Read the model definition and answer for the solid it produces. Units are mm, in the model's axes. A direction names the side the tool comes from. Coordinates: 2 decimals unless noted, no trailing zeros. Order: outer loops, then holes, each group sorted by start corner. A loop starts at its lowest first (then second) coordinate and runs counter-clockwise, first axis right, second up. Notation, with made-up numbers: M -4.5,82.25 L 46.5,82.25 A13 cw 46.5,101.25 Z; hole C 0.25,77.5 d6. An arc over 180 degrees is marked long. Write each question's results on one line, items separated by ' | '.
```python
from build123d import *

# Parameters (mm, degrees)
F1_DEPTH     = 25.4
F3_DEPTH     = 25.401
F4_T1_DEPTH  = 75.1590131963
F4_T6_DEPTH  = 127
F4_T11_DEPTH = 127
F4_T16_DEPTH = 127
F4_T21_DEPTH = 127
F4_T26_DEPTH = 121.344223221
F4_T31_DEPTH = 121.344223221
F4_T36_DEPTH = 121.344223221
F4_T41_DEPTH = 121.344223221
F4_T47_DEPTH = 121.344223221
F4_T51_DEPTH = 127
F4_T58_DEPTH = 127
F4_T62_DEPTH = 121.344223221
F4_T69_DEPTH = 121.344223221
F4_T73_DEPTH = 127
F4_T80_DEPTH = 127
F4_T84_DEPTH = 121.344223221


# Not quite as in the source:
# - a fillet or chamfer that OpenCascade refuses, or shapes differently, is made with other operations: its cross-section is extruded or revolved along the edge and cut away or added


with BuildPart() as f1:
    # F0 (on Front) → F1 (new body)
    with BuildSketch(Plane.XZ):
        Polygon((4.8083475167, 0), (0, 0), (-4.8083475167, 0), (-50.8, 63.5), (-68.9793676138, 63.5), (-12.7, -14.2040973853), (-12.7, -115.8040973853), (0, -115.8040973853), (12.7, -115.8040973853), (12.7, -14.2040973853), (68.9793676138, 63.5), (50.8, 63.5), align=None)
    extrude(amount=F1_DEPTH)

    # F2 (on face) → F3 (cut, through all)
    with BuildSketch(Plane(origin=(0, 0, 0), x_dir=(-1, 0, 0), z_dir=(0, 1, 0))):
        with BuildLine():
            ThreePointArc((-46.3238090676, 51.3453096211), (-51.0863090676, 56.1078096211), (-55.8488090676, 51.3453096211))
            Line((-55.8488090676, 51.3453096211), (-46.3238090676, 51.3453096211))
        make_face()
        with BuildLine():
            Line((-46.3238090676, 51.3453096211), (-55.8488090676, 51.3453096211))
            ThreePointArc((-55.8488090676, 51.3453096211), (-51.0863090676, 46.5828096211), (-46.3238090676, 51.3453096211))
        make_face()
        with BuildLine():
            ThreePointArc((55.8488090676, 51.3453096211), (51.0863090676, 56.1078096211), (46.3238090676, 51.3453096211))
            Line((46.3238090676, 51.3453096211), (55.8488090676, 51.3453096211))
        make_face()
        with BuildLine():
            Line((55.8488090676, 51.3453096211), (46.3238090676, 51.3453096211))
            ThreePointArc((46.3238090676, 51.3453096211), (51.0863090676, 46.5828096211), (55.8488090676, 51.3453096211))
        make_face()
    extrude(amount=-F3_DEPTH, mode=Mode.SUBTRACT)

    # F4: fillet of radius 5.08 on 10 edges, made by hand

    # F4_s2 → F4_t1 (cut)
    with BuildSketch(Plane.XZ.offset(-24.8795065982)):
        with BuildLine():
            ThreePointArc((-63.1417971968, 55.440152148), (-63.552165901, 60.7296290732), (-59.0275649745, 63.5))
            Line((-59.0275649745, 63.5), (-68.9793676138, 63.5))
            Line((-68.9793676138, 63.5), (-63.1417971968, 55.440152148))
        make_face()
        with BuildLine():
            ThreePointArc((63.1417971968, 55.440152148), (63.552165901, 60.7296290732), (59.0275649745, 63.5))
            Line((59.0275649745, 63.5), (68.9793676138, 63.5))
            Line((68.9793676138, 63.5), (63.1417971968, 55.440152148))
        make_face()
    extrude(amount=F4_T1_DEPTH, mode=Mode.SUBTRACT)


with BuildPart() as f4_tool4:
    # F4_s5 → F4_t6 (new body)
    with BuildSketch(Plane.XY.offset(-128.5040973853)):
        with BuildLine():
            ThreePointArc((12.7, -5.08), (11.2121024484, -1.4878975516), (7.62, 0))
            Line((7.62, 0), (12.7, 0))
            Line((12.7, 0), (12.7, -5.08))
        make_face()
    extrude(amount=F4_T6_DEPTH)

    split(bisect_by=Plane(origin=(15.0780779602, 0, -10.9207200262), x_dir=(0, 1, 0), z_dir=(0.8098882327, 0, -0.5865842228)), keep=Keep.TOP)


with BuildPart() as f1_1:
    add(f1.part)

    # F4_t3: cut F4_tool4
    add(f4_tool4.part, mode=Mode.SUBTRACT)


with BuildPart() as f4_tool9:
    # F4_s10 → F4_t11 (new body)
    with BuildSketch(Plane.XY.offset(-1.5040973853)):
        with BuildLine():
            ThreePointArc((-7.62, 0), (-11.2121024484, -1.4878975516), (-12.7, -5.08))
            Line((-12.7, -5.08), (-12.7, 0))
            Line((-12.7, 0), (-7.62, 0))
        make_face()
    extrude(amount=-F4_T11_DEPTH)

    split(bisect_by=Plane(origin=(-15.0780779602, 0, -10.9207200262), x_dir=(0, 1, 0), z_dir=(-0.8098882327, 0, -0.5865842228)), keep=Keep.TOP)


with BuildPart() as f1_2:
    add(f1_1.part)

    # F4_t8: cut F4_tool9
    add(f4_tool9.part, mode=Mode.SUBTRACT)


with BuildPart() as f4_tool14:
    # F4_s15 → F4_t16 (new body)
    with BuildSketch(Plane.XY.offset(-128.5040973853)):
        with BuildLine():
            ThreePointArc((12.7, -20.32), (11.2121024484, -23.9121024484), (7.62, -25.4))
            Line((7.62, -25.4), (12.7, -25.4))
            Line((12.7, -25.4), (12.7, -20.32))
        make_face()
    extrude(amount=F4_T16_DEPTH)

    split(bisect_by=Plane(origin=(15.0780779602, 0, -10.9207200262), x_dir=(0, 1, 0), z_dir=(0.8098882327, 0, -0.5865842228)), keep=Keep.TOP)


with BuildPart() as f1_3:
    add(f1_2.part)

    # F4_t13: cut F4_tool14
    add(f4_tool14.part, mode=Mode.SUBTRACT)


with BuildPart() as f4_tool19:
    # F4_s20 → F4_t21 (new body)
    with BuildSketch(Plane.XY.offset(-1.5040973853)):
        with BuildLine():
            ThreePointArc((-7.62, -25.4), (-11.2121024484, -23.9121024484), (-12.7, -20.32))
            Line((-12.7, -20.32), (-12.7, -25.4))
            Line((-12.7, -25.4), (-7.62, -25.4))
        make_face()
    extrude(amount=-F4_T21_DEPTH)

    split(bisect_by=Plane(origin=(-15.0780779602, 0, -10.9207200262), x_dir=(0, 1, 0), z_dir=(-0.8098882327, 0, -0.5865842228)), keep=Keep.TOP)


with BuildPart() as f1_4:
    add(f1_3.part)

    # F4_t18: cut F4_tool19
    add(f4_tool19.part, mode=Mode.SUBTRACT)


with BuildPart() as f4_tool24:
    # F4_s25 → F4_t26 (new body)
    with BuildSketch(Plane(origin=(-9.8276975902, 0, -13.5689579148), x_dir=(0, 1, 0), z_dir=(0.5865842228, 0, 0.8098882327))):
        with BuildLine():
            ThreePointArc((-20.32, -18.6174799816), (-23.9121024484, -17.12958243), (-25.4, -13.5374799816))
            Line((-25.4, -13.5374799816), (-25.4, -18.6174799816))
            Line((-25.4, -18.6174799816), (-20.32, -18.6174799816))
        make_face()
    extrude(amount=F4_T26_DEPTH)

    split(bisect_by=Plane.YZ.offset(12.7), keep=Keep.TOP)


with BuildPart() as f1_5:
    add(f1_4.part)

    # F4_t23: cut F4_tool24
    add(f4_tool24.part, mode=Mode.SUBTRACT)


with BuildPart() as f4_tool29:
    # F4_s30 → F4_t31 (new body)
    with BuildSketch(Plane(origin=(-9.8276975902, 0, -13.5689579148), x_dir=(0, 1, 0), z_dir=(0.5865842228, 0, 0.8098882327))):
        with BuildLine():
            ThreePointArc((-5.08, -18.6174799816), (-1.4878975516, -17.12958243), (0, -13.5374799816))
            Line((0, -13.5374799816), (0, -18.6174799816))
            Line((0, -18.6174799816), (-5.08, -18.6174799816))
        make_face()
    extrude(amount=F4_T31_DEPTH)

    split(bisect_by=Plane.YZ.offset(12.7), keep=Keep.TOP)


with BuildPart() as f1_6:
    add(f1_5.part)

    # F4_t28: cut F4_tool29
    add(f4_tool29.part, mode=Mode.SUBTRACT)


with BuildPart() as f4_tool34:
    # F4_s35 → F4_t36 (new body)
    with BuildSketch(Plane(origin=(-61.3509092836, 0, 84.7063005819), x_dir=(0, 1, 0), z_dir=(0.5865842228, 0, -0.8098882327))):
        with BuildLine():
            ThreePointArc((-25.4, -13.5374799816), (-23.9121024484, -17.12958243), (-20.32, -18.6174799816))
            Line((-20.32, -18.6174799816), (-25.4, -18.6174799816))
            Line((-25.4, -18.6174799816), (-25.4, -13.5374799816))
        make_face()
    extrude(amount=F4_T36_DEPTH)

    split(bisect_by=Plane.YZ.offset(-12.7), keep=Keep.BOTTOM)


with BuildPart() as f1_7:
    add(f1_6.part)

    # F4_t33: cut F4_tool34
    add(f4_tool34.part, mode=Mode.SUBTRACT)


with BuildPart() as f4_tool39:
    # F4_s40 → F4_t41 (new body)
    with BuildSketch(Plane(origin=(-61.3509092836, 0, 84.7063005819), x_dir=(0, 1, 0), z_dir=(0.5865842228, 0, -0.8098882327))):
        with BuildLine():
            ThreePointArc((0, -13.5374799816), (-1.4878975516, -17.12958243), (-5.08, -18.6174799816))
            Line((-5.08, -18.6174799816), (0, -18.6174799816))
            Line((0, -18.6174799816), (0, -13.5374799816))
        make_face()
    extrude(amount=F4_T41_DEPTH)

    split(bisect_by=Plane.YZ.offset(-12.7), keep=Keep.BOTTOM)


with BuildPart() as f1_8:
    add(f1_7.part)

    # F4_t38: cut F4_tool39
    add(f4_tool39.part, mode=Mode.SUBTRACT)


with BuildPart() as f4_tool45:
    # F4_s46 → F4_t47 (new body)
    with BuildSketch(Plane(origin=(-9.8276975902, 0, -13.5689579148), x_dir=(0, 1, 0), z_dir=(0.5865842228, 0, 0.8098882327))):
        with BuildLine():
            ThreePointArc((-5.08, -18.6174799816), (-1.4878975516, -17.12958243), (0, -13.5374799816))
            Line((0, -13.5374799816), (0, -18.6174799816))
            Line((0, -18.6174799816), (-5.08, -18.6174799816))
        make_face()
    extrude(amount=F4_T47_DEPTH)

    split(bisect_by=Plane.YZ.offset(12.7), keep=Keep.BOTTOM)


with BuildPart() as f4_tool49:
    # F4_s50 → F4_t51 (new body)
    with BuildSketch(Plane.XY.offset(-128.5040973853)):
        with BuildLine():
            ThreePointArc((12.7, -5.08), (11.2121024484, -1.4878975516), (7.62, 0))
            Line((7.62, 0), (12.7, 0))
            Line((12.7, 0), (12.7, -5.08))
        make_face()
    extrude(amount=F4_T51_DEPTH)

    split(bisect_by=Plane(origin=(15.0780779602, 0, -10.9207200262), x_dir=(0, 1, 0), z_dir=(-0.8098882327, 0, 0.5865842228)), keep=Keep.TOP)


with BuildPart() as f4_tool45_1:
    add(f4_tool45.part)

    # F4_t53: intersect F4_tool49
    add(f4_tool49.part, mode=Mode.INTERSECT)


with BuildPart() as f1_9:
    add(f1_8.part)

    # F4_t43: cut F4_tool45
    add(f4_tool45_1.part, mode=Mode.SUBTRACT)


with BuildPart() as f4_tool56:
    # F4_s57 → F4_t58 (new body)
    with BuildSketch(Plane.XY.offset(-1.5040973853)):
        with BuildLine():
            ThreePointArc((-7.62, 0), (-11.2121024484, -1.4878975516), (-12.7, -5.08))
            Line((-12.7, -5.08), (-12.7, 0))
            Line((-12.7, 0), (-7.62, 0))
        make_face()
    extrude(amount=-F4_T58_DEPTH)

    split(bisect_by=Plane(origin=(-15.0780779602, 0, -10.9207200262), x_dir=(0, 1, 0), z_dir=(0.8098882327, 0, 0.5865842228)), keep=Keep.TOP)


with BuildPart() as f4_tool60:
    # F4_s61 → F4_t62 (new body)
    with BuildSketch(Plane(origin=(-61.3509092836, 0, 84.7063005819), x_dir=(0, 1, 0), z_dir=(0.5865842228, 0, -0.8098882327))):
        with BuildLine():
            ThreePointArc((0, -13.5374799816), (-1.4878975516, -17.12958243), (-5.08, -18.6174799816))
            Line((-5.08, -18.6174799816), (0, -18.6174799816))
            Line((0, -18.6174799816), (0, -13.5374799816))
        make_face()
    extrude(amount=F4_T62_DEPTH)

    split(bisect_by=Plane.YZ.offset(-12.7), keep=Keep.TOP)


with BuildPart() as f4_tool56_1:
    add(f4_tool56.part)

    # F4_t64: intersect F4_tool60
    add(f4_tool60.part, mode=Mode.INTERSECT)


with BuildPart() as f1_10:
    add(f1_9.part)

    # F4_t54: cut F4_tool56
    add(f4_tool56_1.part, mode=Mode.SUBTRACT)


with BuildPart() as f4_tool67:
    # F4_s68 → F4_t69 (new body)
    with BuildSketch(Plane(origin=(-9.8276975902, 0, -13.5689579148), x_dir=(0, 1, 0), z_dir=(0.5865842228, 0, 0.8098882327))):
        with BuildLine():
            ThreePointArc((-20.32, -18.6174799816), (-23.9121024484, -17.12958243), (-25.4, -13.5374799816))
            Line((-25.4, -13.5374799816), (-25.4, -18.6174799816))
            Line((-25.4, -18.6174799816), (-20.32, -18.6174799816))
        make_face()
    extrude(amount=F4_T69_DEPTH)

    split(bisect_by=Plane.YZ.offset(12.7), keep=Keep.BOTTOM)


with BuildPart() as f4_tool71:
    # F4_s72 → F4_t73 (new body)
    with BuildSketch(Plane.XY.offset(-128.5040973853)):
        with BuildLine():
            ThreePointArc((12.7, -20.32), (11.2121024484, -23.9121024484), (7.62, -25.4))
            Line((7.62, -25.4), (12.7, -25.4))
            Line((12.7, -25.4), (12.7, -20.32))
        make_face()
    extrude(amount=F4_T73_DEPTH)

    split(bisect_by=Plane(origin=(15.0780779602, 0, -10.9207200262), x_dir=(0, 1, 0), z_dir=(-0.8098882327, 0, 0.5865842228)), keep=Keep.TOP)


with BuildPart() as f4_tool67_1:
    add(f4_tool67.part)

    # F4_t75: intersect F4_tool71
    add(f4_tool71.part, mode=Mode.INTERSECT)


with BuildPart() as f1_11:
    add(f1_10.part)

    # F4_t65: cut F4_tool67
    add(f4_tool67_1.part, mode=Mode.SUBTRACT)


with BuildPart() as f4_tool78:
    # F4_s79 → F4_t80 (new body)
    with BuildSketch(Plane.XY.offset(-1.5040973853)):
        with BuildLine():
            ThreePointArc((-7.62, -25.4), (-11.2121024484, -23.9121024484), (-12.7, -20.32))
            Line((-12.7, -20.32), (-12.7, -25.4))
            Line((-12.7, -25.4), (-7.62, -25.4))
        make_face()
    extrude(amount=-F4_T80_DEPTH)

    split(bisect_by=Plane(origin=(-15.0780779602, 0, -10.9207200262), x_dir=(0, 1, 0), z_dir=(0.8098882327, 0, 0.5865842228)), keep=Keep.TOP)


with BuildPart() as f4_tool82:
    # F4_s83 → F4_t84 (new body)
    with BuildSketch(Plane(origin=(-61.3509092836, 0, 84.7063005819), x_dir=(0, 1, 0), z_dir=(0.5865842228, 0, -0.8098882327))):
        with BuildLine():
            ThreePointArc((-25.4, -13.5374799816), (-23.9121024484, -17.12958243), (-20.32, -18.6174799816))
            Line((-20.32, -18.6174799816), (-25.4, -18.6174799816))
            Line((-25.4, -18.6174799816), (-25.4, -13.5374799816))
        make_face()
    extrude(amount=F4_T84_DEPTH)

    split(bisect_by=Plane.YZ.offset(-12.7), keep=Keep.TOP)


with BuildPart() as f4_tool78_1:
    add(f4_tool78.part)

    # F4_t86: intersect F4_tool82
    add(f4_tool82.part, mode=Mode.INTERSECT)


with BuildPart() as f1_12:
    add(f1_11.part)

    # F4_t76: cut F4_tool78
    add(f4_tool78_1.part, mode=Mode.SUBTRACT)


solid = f1_12.part
```
(1) The part is cut by section A-A, the plane y = -9. Write down the section's boundary in (x, z) (1 decimal).
Conclusion:
outline: M -63.1,55.4 L -12.7,-14.2 L -12.7,-115.8 L 12.7,-115.8 L 12.7,-14.2 L 63.1,55.4 A5.1 ccw 59,63.5 L 50.8,63.5 L 4.8,0 L -4.8,0 L -50.8,63.5 L -59,63.5 A5.1 ccw Z; hole C -51.1,51.3 d9.5; hole C 51.1,51.3 d9.5
(2) The part is cut by section B-B, the plane x = -2.5. Write down the section's boundary in (y, z).
Conclusion:
outline: M -25.4,-115.8 L 0,-115.8 L 0,0 L -25.4,0 Z
(3) Straight lines are drawn through the part: line 1 (X direction, y = -12.25, z = -103); line 2 (X direction, y = -12.5, z = 15.5); line 3 (X direction, y = -15.5, z = 5.5). For each, find the intervals that lie inside material, in ascending order.
Conclusion:
line 1: -12.7 to 12.7 | line 2: -34.21 to -16.03, 16.03 to 34.21 | line 3: -26.97 to -8.79, 8.79 to 26.97
(4) For faces 4 (the flat face through (-12.7, -13, -64)), 5 (the flat face through (12.7, -13, -66)), 6 (the cylindrical face through (11.251, -23.872, -64.904)), 7 (the flat face through (28.126, -12.522, 32.194)), determine the directions among +Z, -Z, +X, -X, +Y, -Y from which every point of the face is accessible in a straight line to the end or side of a thin tool.
Conclusion:
face 4: -Z, -X, +Y, -Y | face 5: -Z, +X, +Y, -Y | face 6: -Z, +X, -Y | face 7: +Z, +Y, -Y
(5) The mould has two halves that part along Z. Classify faces 1 (the cylindrical face through (-11.172, -23.951, -63.458)), 2 (the flat face through (0, -13, -115.804)), 3 (the cylindrical face through (-52.1, -12.5, 56)): pulls with the +Z half, pulls with the -Z half, needs draft (parallel to the pull), parting line crosses it, or undercut.
Conclusion:
face 1: needs draft | face 2: pulls with the -Z half | face 3: undercut
(6) Given pin 1 (12 mm diameter, centred on y = -9, z = -40, fed in from -X); pin 2 (3 mm diameter, centred on x = -1.5, y = -14, fed in from +Z); pin 3 (8 mm diameter, centred on x = 23, y = -4.5, fed in from +Z); pin 4 (12 mm diameter, centred on x = -20.5, z = 34, fed in from +Y), each flat-ended and moving along its own axis, determine where each tip first touches the part or whether it passes through.
Conclusion:
pin 1: x = -12.7 | pin 2: z = 0 | pin 3: z = 30.64 | pin 4: through
